Geometry: see drawing. Coordinates: mm, zero at the bounding-box minimum. A direction names the side the tool comes from. Give positions to 0.01 mm unless a question says otherwise; leave off trailing zeros. Loops run counter-clockwise (first coordinate to the right, second up) from the corner with the lowest first, then second, coordinate; pieces in that order, holes last. Notation, with made-up numbers: (23.5, -8.5) -> (69.5, -8.5) arc R24 cw to (69.5, 9.5) -> close; hole circle Ø2 at (21, 85). An arc over 180 degrees is marked (long way). Return JSON: item names as keys, results as strings. Group by question number.
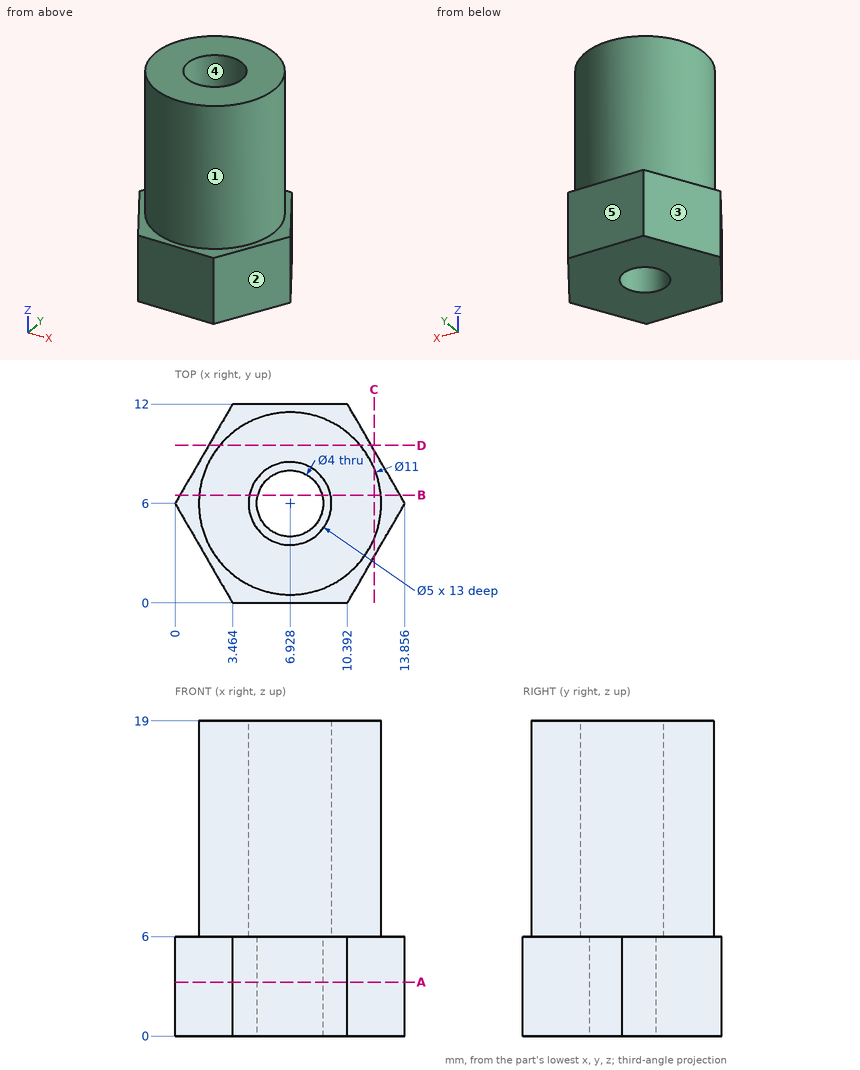
1) Cut plane D-D on y = 9.5. Return loops of the section in (x, z) (1 decimal), then the cut area to 3 significant figures.
2) Contact query for flat-ended pins moving along their axis: P1, Ø6, axis at x = 9, y = 5.5, coming from the +Z side; P2, Ø1, axis at y = 1.5, z = 3, coming from the +X side; P3, Ø6, axis at x = 4.5, z = 11.5, coming from the +Y side; P4, Ø1.5, axis at y = 1.5, z = 11.5, coming from the +X side. Output: stop coordinate, or through.
3) Cut plane C-C on x = 12. Return loops of the section in (y, z) (1 decimal).
4) Mould query, pull axis X, two halves, no side actions, for the marked faces 3, 4 and 5. Classes: released by +X, released by -X, zero draft, split by the parting line, or undercut.
5) Cut plane B-B on y = 6.5. Return loops of the section in (x, z) (1 decimal), then the cut area to 3 significant figures.
6) Cut plane A-A on z = 3.25. Return loops of the section in (x, y).
7) Reachability of the marked faces 1 and 2 from +Z, -Z, +X, -X, +Y, -Y: full face, straight path, thin tool, end or side. Return the list, or none.
8) Material intervals for line 1 (Z direction, x = 10.5, y = 11); line 2 (Y direction, x = 8.25, z = 3.25); line 3 (Y direction, x = 7.25, z = 4.75) (1 decimal), sorted ascending.
Calculated:
{
 "1": {"outline": "(2, 0) -> (11.8, 0) -> (11.8, 6) -> (11.2, 6) -> (11.2, 19) -> (2.7, 19) -> (2.7, 6) -> (2, 6) -> close", "area": "169 mm2"},
 "2": {"P1": "z = 19", "P2": "x = 11.55", "P3": "y = 11.5", "P4": "x = 10.95"},
 "3": {"outline": "(2.8, 0) -> (9.2, 0) -> (9.2, 6) -> (8.1, 6) -> (8.1, 19) -> (3.9, 19) -> (3.9, 6) -> (2.8, 6) -> close"},
 "4": {"face 3": "released by -X", "face 4": "undercut", "face 5": "zero draft"},
 "5": {"outline": "(0.3, 0) -> (5, 0) -> (5, 6) -> (4.5, 6) -> (4.5, 19) -> (1.5, 19) -> (1.5, 6) -> (0.3, 6) -> close; (8.9, 0) -> (13.6, 0) -> (13.6, 6) -> (12.4, 6) -> (12.4, 19) -> (9.4, 19) -> (9.4, 6) -> (8.9, 6) -> close", "area": "135 mm2"},
 "6": {"outline": "(0, 6) -> (3.46, 0) -> (10.39, 0) -> (13.86, 6) -> (10.39, 12) -> (3.46, 12) -> close; hole circle Ø4 at (6.93, 6)"},
 "7": {"face 1": "+Z", "face 2": "+Z, -Z, +X, -Y"},
 "8": {"line 1": "0 to 6", "line 2": "0 to 4.5, 7.5 to 12", "line 3": "0 to 4, 8 to 12"}
}
